For this review, take the finished solid that the model builds, in its own axes (mm). Coordinates: 2 decimals unless noted, no trailing zeros. Loops run counter-clockwise (first coordinate to the right, second up) from the corner with the lowest first, then second, coordinate; pieces in that order, holes last. Notation, with made-up numbers: M -29.5,78 L 14.5,78 A16 ccw 14.5,109 Z; hole C 45.5,-31.5 d1. An arc over 180 degrees is marked long. Write item = value, one per line.
from build123d import *

# Parameters (mm, degrees)
F0_W     = 76.2
F0_H     = 48.466104
F1_DEPTH = 25.4
F2_R     = 15


with BuildPart() as f1:
    # F0 (on Front) → F1 (new body)
    with BuildSketch(Plane.XZ):
        Rectangle(F0_W, F0_H)
    extrude(amount=F1_DEPTH)

    # F2 (on face) → F3 (revolve, cut)
    with BuildSketch(Plane.XZ):
        Circle(F2_R)
    revolve(axis=Axis((0, 0, -24.233052), (-1, 0, 0)), mode=Mode.SUBTRACT)


solid = f1.part
Q1. For line 1 along X through (y, z) = (-14.5, 1.5); line 2 along X through (y, z) = (-6, -11.5); line 3 along Z through (x, y) = (11.5, -3), list the stretches that pass through material, from the lowest coordinate up.
Solved:
line_1 = -38.1 to -14.03, 14.03 to 38.1
line_2 = -38.1 to -11.04, 11.04 to 38.1
line_3 = -24.23 to -9.94, 9.5 to 24.23
Q2. For pin 1 Ø5 at (x, y) = (12, -16.5) entering from -Z, flat-tipped, find the tip position at first contact; note if it passes through.
Solved:
pin_1 = -24.23
Q3. Add section A-A (x = 0.5). Write out the cut boundary in (y, z).
Solved:
outline = M -25.4,5.66 A39.22 cw 0,14.99 L 0,24.23 L -25.4,24.23 Z; M -9.24,-24.23 L 0,-24.23 L 0,-14.99 A9.24 ccw Z
